Autodesk Inventor part; units mm, degrees
ref_plane "YZ Plane" through (0, 0, 0) normal (1, 0, 0) x (0, 1, 0)
ref_plane "XZ Plane" through (0, 0, 0) normal (0, 1, 0) x (-1, 0, 0)
ref_plane "XY Plane" through (0, 0, 0) normal (0, 0, 1) x (1, 0, 0)
sketch "草圖1" plane through (0, 0, 0) normal (0, 1, 0) x (-1, 0, 0)
  line L0 (4.4578, 4.5382) -> (-8.0422, 4.5382)
  line L1 (-8.0422, 4.5382) -> (-8.0422, -5.4618)
  line L2 (-8.0422, -5.4618) -> (4.4578, -5.4618)
  line L3 (4.4578, -5.4618) -> (4.4578, 4.5382)
  line L4 (5.4578, -6.4618) -> (-9.0422, -6.4618)
  line L5 (-9.0422, -6.4618) -> (-9.0422, 5.5382)
  line L6 (-9.0422, 5.5382) -> (5.4578, 5.5382)
  line L7 (5.4578, 5.5382) -> (5.4578, -6.4618)
  point P0 (0, 0)
  dimension "d0" = 10
  dimension "d1" = 12.5
  dimension "d2" = 1
extrude "擠出1" add sketch "草圖1" along normal blind 20
properties part number "axis_rf_fix"
The model under review builds one solid part; all positions refer to its coordinate system, in mm. A direction names the side the tool comes from. Round coordinates to 2 decimals unless told otherwise and drop trailing zeros. Write each loop counter-clockwise with the first axis right and the second up, starting at its lowest first coordinate (ties: lowest second). Pieces come first, ordered by that corner, then holes. Notation, with made-up numbers: (-33, -10) - (-8, -10) arc R19 ccw to (-8, -1) - close; hole circle Ø9 at (74.25, 7.25). An arc over 180 degrees is marked (long way). Answer as CSV lines item,"result". Start each with the question number.
(1) For pin 1 Ø1.5 at (x, z) = (7, -3.5) entering from -Y, flat-tipped, find the tip position at first contact; note if it passes through.
(2) For faces 1 (the flat face through (2, 10, -6.462)), 2 (the flat face through (2, 10, 4.538)), list the 3-axis set-ups (+Z, -Z, +X, -X, +Y, -Y) from which the entire face can be reached by the end or side of a thin tool; tool diameter is ignored.
(3) We need section C-C on y = 9. State the section outline as (x, z) points.
(4) We need section A-A on x = -1.5. State the section outline as (y, z) points.
(5) We need section B-B on z = 0.75. State the section outline as (x, y) points, plus the area to 3 significant figures.
(6) Draft analysis for pull direction X (two halves, no side actions). For faces 3 (the flat face through (9.042, 10, -1)), 4 (the flat face through (8.042, 10, 0)), 5 (the flat face through (2, 10, 5.538)), state which applies: pulls with the +X half, pulls with the -X half, needs draft (parallel to the pull), parting line crosses it, or undercut.
(7) To check wall thickness, follow line 1 (Z direction, x = 5.5, y = 3.5); line 2 (X direction, y = 4.5, z = 0.5). State the ranges of each line that lie inside material, in increasing order.
Worked answers:
1,pin 1,"through"
2,face 1,"-Z, +X, -X, +Y, -Y"
2,face 2,"+Y, -Y"
3,outline,"(-5.46, -6.46) - (9.04, -6.46) - (9.04, 5.54) - (-5.46, 5.54) - close; hole (-4.46, -5.46) - (8.04, -5.46) - (8.04, 4.54) - (-4.46, 4.54) - close"
4,outline,"(0, -6.46) - (20, -6.46) - (20, -5.46) - (0, -5.46) - close; (0, 4.54) - (20, 4.54) - (20, 5.54) - (0, 5.54) - close"
5,outline,"(-5.46, 0) - (-4.46, 0) - (-4.46, 20) - (-5.46, 20) - close; (8.04, 0) - (9.04, 0) - (9.04, 20) - (8.04, 20) - close"
5,area,"40.0 mm²"
6,face 3,"pulls with the +X half"
6,face 4,"undercut"
6,face 5,"needs draft"
7,line 1,"-6.46 to -5.46, 4.54 to 5.54"
7,line 2,"-5.46 to -4.46, 8.04 to 9.04"
